Input: part model. Units: mm. Frame: model coordinates. Face numbers are marked on the shaded views. Round coordinates to 2 decimals unless told otherwise and drop trailing zeros. Order: outer loops, then holes, each group sorted by start corner. A loop starts at its lowest first (then second) coordinate and runs counter-clockwise, first axis right, second up.
Item 1: Mould query, pull axis X, two halves, no side actions, for the marked faces 1 and 2. Classes: released by +X, released by -X, zero draft, split by the parting line, or undercut.
Item 2: Cut plane C-C on x = -175. Output: boundary loops of the cut face in (y, z).
Item 3: Cut plane B-B on z = 25. Output: boundary loops of the cut face in (x, y), then the cut area to 3 significant figures.
Item 4: Cut plane A-A on y = -1.4. Output: boundary loops of the cut face in (x, z), then the cut area to 3 significant figures.
Item 5: Cut plane D-D on z = 35. Output: boundary loops of the cut face in (x, y), then the cut area to 3 significant figures.
Item 6: Line query: L1, parallel to Z at x = -175, y = -1.95; L2, parallel to Z at x = -100, y = -1.9; L3, parallel to X at y = -1.6, z = 22. Output: solid intervals per line, ascending.
Item 7: First-contact query: pin 1 (1 mm diameter, centred on x = -34.5, y = -1, fed in from -Z); pin 2 (25 mm diameter, centred on x = -135, z = 27.5, fed in from -Y). Flat tips, straight axial feed; report the tip coordinate or a pass-through.
Autodesk Inventor part; units mm, degrees
ref_plane "YZ Plane" through (0, 0, 0) normal (1, 0, 0) x (0, 1, 0)
ref_plane "XZ Plane" through (0, 0, 0) normal (0, 1, 0) x (-1, 0, 0)
ref_plane "XY Plane" through (0, 0, 0) normal (0, 0, 1) x (1, 0, 0)
sketch "Sketch1" plane through (0, 0, 0) normal (0, 1, 0) x (-1, 0, 0)
  line L0 (0, 0) -> (200, 0)
  line L1 (200, 0) -> (200, 50)
  line L2 (200, 50) -> (0, 50)
  line L3 (0, 50) -> (0, 0)
  line L4 (100, 50) -> (100, -12.2978) construction
  line L5 (100, 46.202) -> (25, 46.202) construction
  line L6 (25, 46.202) -> (25, 4.511) construction
  line L7 (14.6583, 50) -> (14.6583, 25) construction
  line L8 (14.6583, 25) -> (197.0399, 25) construction
  line L9 (110.8785, 50) -> (110.8785, 35) construction
  line L10 (110.8785, 35) -> (88.7756, 35) construction
  dimension "d0" = 200
  dimension "d1" = 50
  dimension "d2" = 75
  dimension "d3" = 25
  dimension "d4" = 15
extrude "Extrusion1" add sketch "Sketch1" along normal blind 3
sketch "Sketch2" plane through (0, 0, 0) normal (0, -1, 0) x (1, 0, 0)
  line L0 (0, 0) -> (-200, 0)
  line L1 (-200, 50) -> (0, 50)
  line L2 (-200, 0) -> (-200, 50)
  line L3 (-100, 50) -> (-100, -20.2581) construction
  line L4 (-200, 25) -> (-5.0979, 25) construction
  line L5 (-100, 50) -> (-100, 35) construction
  line L6 (-100, 35) -> (-80.8703, 35) construction
  line L7 (-100, 35) -> (-119.3164, 35) construction
  line L8 (-190.2363, 50) -> (-190.2363, 25) construction
  line L9 (-100, 0) -> (-175, 0) construction
  line L10 (-175, 0) -> (-175, 41.5169) construction
  line L11 (-100, 0) -> (-25, 0) construction
  line L12 (-25, 0) -> (-25, 41.5169) construction
  circle A0 centre (-100, 35) radius 4
  circle A1 centre (-100, 35) radius 6
  dimension "d7" = 15
  dimension "d8" = 25
  dimension "d9" = 75
  dimension "d10" = 75
  dimension "d11" = 8
  dimension "d12" = 12
extrude "Extrusion2" add sketch "Sketch2" along normal blind 3
sketch "Sketch3" plane through (0, 0, 0) normal (0, -1, 0) x (1, 0, 0)
  line L0 (-200, 50) -> (0, 50)
  line L1 (-200, 0) -> (-200, 50)
  circle A0 centre (-100, 35) radius 6
  line L2 (-100, 35) -> (-175, 35) construction
  line L3 (-175, 35) -> (-175, -16.3605) construction
  line L4 (-191.9526, 50) -> (-191.9526, 25) construction
  line L5 (-191.9526, 25) -> (-42.7931, 25) construction
  circle A1 centre (-175, 25) radius 5
  circle A2 centre (-175, 25) radius 7
  dimension "d15" = 75
  dimension "d16" = 25
  dimension "d17" = 10
  dimension "d18" = 14
extrude "Extrusion3" add sketch "Sketch3" along normal blind 3 contours A2
sketch "Sketch4" plane through (0, 0, 0) normal (0, -1, 0) x (1, 0, 0)
  circle A0 centre (-100, 35) radius 6
  line L0 (-200, 50) -> (0, 50)
  line L1 (-200, 0) -> (-200, 50)
  line L2 (-100, 35) -> (-25, 35) construction
  line L3 (-25, 35) -> (-25, -20.2088) construction
  line L4 (-14.8647, 50) -> (-14.8647, 25) construction
  line L5 (-14.8647, 25) -> (-71.3929, 25) construction
  circle A1 centre (-25, 25) radius 5
  circle A2 centre (-25, 25) radius 7
  dimension "d21" = 75
  dimension "d22" = 25
  dimension "d23" = 10
  dimension "d24" = 14
extrude "Extrusion4" add sketch "Sketch4" along normal blind 3 contours A2
properties part number "z rods top bracket"
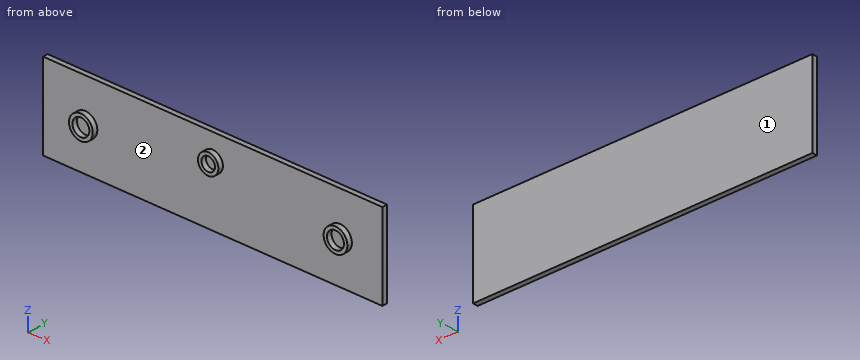
From the geometry:
1. face 1: zero draft
1. face 2: undercut
2. outline: (-3, 18) - (0, 18) - (0, 0) - (3, 0) - (3, 50) - (0, 50) - (0, 32) - (-3, 32) - (-3, 30) - (0, 30) - (0, 20) - (-3, 20) - close
3. outline: (-200, 0) - (-182, 0) - (-182, -3) - (-180, -3) - (-180, 0) - (-170, 0) - (-170, -3) - (-168, -3) - (-168, 0) - (-32, 0) - (-32, -3) - (-30, -3) - (-30, 0) - (-20, 0) - (-20, -3) - (-18, -3) - (-18, 0) - (0, 0) - (0, 3) - (-200, 3) - close
3. area: 624 mm2
4. outline: circle Ø14 at (-175, 25); circle Ø12 at (-100, 35); circle Ø14 at (-25, 25); hole circle Ø10 at (-175, 25); hole circle Ø8 at (-100, 35); hole circle Ø10 at (-25, 25)
4. area: 214 mm2
5. outline: (-200, 0) - (-106, 0) - (-106, -3) - (-104, -3) - (-104, 0) - (-96, 0) - (-96, -3) - (-94, -3) - (-94, 0) - (0, 0) - (0, 3) - (-200, 3) - close
5. area: 612 mm2
6. L1: z = 18 to 20, 30 to 32
6. L2: z = 29 to 31, 39 to 41
6. L3: x = -181.32 to -179, -171 to -168.68, -31.32 to -29, -21 to -18.68
7. pin 1: passes through
7. pin 2: stops at y = 0
